Source: CAD feature listing. Evaluate the final solid. Frame: model axes, mm. A direction names the side the tool comes from. Coordinates: 2 decimals unless noted, no trailing zeros. Order: outer loops, then holes, each group sorted by start corner. A loop starts at its lowest first (then second) coordinate and runs counter-clockwise, first axis right, second up.
```python
from build123d import *

# Parameters (mm, degrees)
SALIENTE_EXTRUIR1_DEPTH = 3


with BuildPart() as part:
    # Croquis1 → Saliente-Extruir1 (new body)
    with BuildSketch(Plane.XY):
        with BuildLine():
            ThreePointArc((-9.805994702, 4.781775998), (-9.445994702, 4.421775998), (-9.445994702, 3.912659116))
            ThreePointArc((-9.445994702, 3.912659116), (-9.805994702, 3.552659116), (-10.315111585, 3.552659116))
            Line((-10.315111585, 3.552659116), (-14.665897198, 5.354813524))
            Line((-14.665897198, 5.354813524), (-14.942220541, 4.584446936))
            ThreePointArc((-14.942220541, 4.584446936), (-13.141116636, 2.599696402), (-12.489358574, 0))
            ThreePointArc((-12.489358574, 0), (-13.40224475, -3.037731981), (-15.838448045, -5.06900997))
            ThreePointArc((-15.838448045, -5.06900997), (-15.725960944, -5.407906335), (-15.606223383, -5.744309383))
            Line((-15.606223383, -5.744309383), (-10.315111585, -3.552659116))
            ThreePointArc((-10.315111585, -3.552659116), (-9.445994702, -3.912659116), (-9.805994702, -4.781775998))
            Line((-9.805994702, -4.781775998), (-15.0971065, -6.973426265))
            ThreePointArc((-15.0971065, -6.973426265), (-14.943900866, -7.295966383), (-14.78380534, -7.615142693))
            ThreePointArc((-14.78380534, -7.615142693), (-9.642639792, -8.161938898), (-7.217280635, -12.727922061))
            ThreePointArc((-7.217280635, -12.727922061), (-7.317660389, -13.774935704), (-7.615142693, -14.78380534))
            ThreePointArc((-7.615142693, -14.78380534), (-7.295966383, -14.943900866), (-6.973426265, -15.0971065))
            Line((-6.973426265, -15.0971065), (-4.781775998, -9.805994702))
            ThreePointArc((-4.781775998, -9.805994702), (-3.912659116, -9.445994702), (-3.552659116, -10.315111585))
            Line((-3.552659116, -10.315111585), (-5.744309383, -15.606223383))
            ThreePointArc((-5.744309383, -15.606223383), (-5.407906335, -15.725960944), (-5.06900997, -15.838448045))
            ThreePointArc((-5.06900997, -15.838448045), (0, -12.489358574), (5.06900997, -15.838448045))
            ThreePointArc((5.06900997, -15.838448045), (5.407906335, -15.725960944), (5.744309383, -15.606223383))
            Line((5.744309383, -15.606223383), (3.552659116, -10.315111585))
            ThreePointArc((3.552659116, -10.315111585), (3.912659116, -9.445994702), (4.781775998, -9.805994702))
            Line((4.781775998, -9.805994702), (6.973426265, -15.0971065))
            ThreePointArc((6.973426265, -15.0971065), (7.295966383, -14.943900866), (7.615142693, -14.78380534))
            ThreePointArc((7.615142693, -14.78380534), (8.83131014, -8.83131014), (14.78380534, -7.615142693))
            ThreePointArc((14.78380534, -7.615142693), (14.943900866, -7.295966383), (15.0971065, -6.973426265))
            Line((15.0971065, -6.973426265), (9.805994702, -4.781775998))
            ThreePointArc((9.805994702, -4.781775998), (9.445994702, -3.912659116), (10.315111585, -3.552659116))
            Line((10.315111585, -3.552659116), (15.606223383, -5.744309383))
            ThreePointArc((15.606223383, -5.744309383), (15.725960944, -5.407906335), (15.838448045, -5.06900997))
            ThreePointArc((15.838448045, -5.06900997), (12.489358574, 0), (15.838448045, 5.06900997))
            ThreePointArc((15.838448045, 5.06900997), (15.725960944, 5.407906335), (15.606223383, 5.744309383))
            Line((15.606223383, 5.744309383), (10.315111585, 3.552659116))
            ThreePointArc((10.315111585, 3.552659116), (9.445994702, 3.912659116), (9.805994702, 4.781775998))
            Line((9.805994702, 4.781775998), (15.0971065, 6.973426265))
            ThreePointArc((15.0971065, 6.973426265), (14.943900866, 7.295966383), (14.78380534, 7.615142693))
            ThreePointArc((14.78380534, 7.615142693), (8.83131014, 8.83131014), (7.615142693, 14.78380534))
            ThreePointArc((7.615142693, 14.78380534), (7.295966383, 14.943900866), (6.973426265, 15.0971065))
            Line((6.973426265, 15.0971065), (4.781775998, 9.805994702))
            ThreePointArc((4.781775998, 9.805994702), (3.912659116, 9.445994702), (3.552659116, 10.315111585))
            Line((3.552659116, 10.315111585), (5.744309383, 15.606223383))
            ThreePointArc((5.744309383, 15.606223383), (5.407906335, 15.725960944), (5.06900997, 15.838448045))
            ThreePointArc((5.06900997, 15.838448045), (0, 12.489358574), (-5.06900997, 15.838448045))
            ThreePointArc((-5.06900997, 15.838448045), (-5.407906335, 15.725960944), (-5.744309383, 15.606223383))
            Line((-5.744309383, 15.606223383), (-3.552659116, 10.315111585))
            ThreePointArc((-3.552659116, 10.315111585), (-3.912659116, 9.445994702), (-4.781775998, 9.805994702))
            Line((-4.781775998, 9.805994702), (-6.973426265, 15.0971065))
            ThreePointArc((-6.973426265, 15.0971065), (-7.295966383, 14.943900866), (-7.615142693, 14.78380534))
            ThreePointArc((-7.615142693, 14.78380534), (-7.317660389, 13.774935704), (-7.217280635, 12.727922061))
            ThreePointArc((-7.217280635, 12.727922061), (-9.642639792, 8.161938898), (-14.78380534, 7.615142693))
            ThreePointArc((-14.78380534, 7.615142693), (-14.870201448, 7.445025684), (-14.954640105, 7.273928642))
            ThreePointArc((-14.954640105, 7.273928642), (-14.628849784, 7.038643274), (-14.422305364, 6.693914482))
            Line((-14.422305364, 6.693914482), (-9.805994702, 4.781775998))
        make_face()
        with BuildLine():
            ThreePointArc((0.665193263, 0), (-0.129772768, -0.652411761), (-0.614558441, 0.254558441))
            ThreePointArc((-0.614558441, 0.254558441), (0.129772768, 0.652411761), (0.665193263, 0))
        make_face(mode=Mode.SUBTRACT)
    extrude(amount=-SALIENTE_EXTRUIR1_DEPTH)


solid = part.part
```
Q1. Material intervals for line 1 along X through (y, z) = (-10.5, -1.95); line 2 along Y through (x, z) = (-5, -2.55); line 3 along Y through (x, z) = (-0.5, -2.05), sorted ascending.
Solutions:
line 1: x = -7.69 to -5.07, -3.63 to 3.63, 5.07 to 7.69
line 2: y = -15.68 to -13.81, -10.33 to 10.33, 13.81 to 15.68
line 3: y = -12.51 to -0.44, 0.44 to 12.51
Q2. Section query B-B on y = -13.5. Output: boundary loops of the cut face in (x, z), plus the area to 3 significant figures.
Solutions:
outline: (-7.27, -3) - (-6.31, -3) - (-6.31, 0) - (-7.27, 0) - close; (-4.87, -3) - (-3.18, -3) - (-3.18, 0) - (-4.87, 0) - close; (3.18, -3) - (4.87, -3) - (4.87, 0) - (3.18, 0) - close; (6.31, -3) - (7.27, -3) - (7.27, 0) - (6.31, 0) - close
area: 15.9 mm2
Q3. Pin query (flat end, axial travel): P1, Ø1.5, axis at x = 3, z = -2, coming from the +Y side; P2, Ø0.8, axis at x = 0, y = 0, coming from the -Z side; P3, Ø1.5, axis at y = -10.5, z = -2.5, coming from the +X side; P4, Ø1, axis at x = -2.5, z = -1.5, coming from the +Y side. Return the tip coordinate at first contact, or that it passes through.
Solutions:
P1: stops at y = 13.96
P2: passes through
P3: stops at x = 8.09
P4: stops at y = 13.38
Q4. Section query A-A on x = 0. Output: boundary loops of the cut face in (y, z).
Solutions:
outline: (-12.49, -3) - (-0.67, -3) - (-0.67, 0) - (-12.49, 0) - close; (0.67, -3) - (12.49, -3) - (12.49, 0) - (0.67, 0) - close
Q5. Set-up query: faces 1 (the flat face through (4.63, 12.92, -1.48)), 2 (the cylindrical face through (-0.09, -12.49, -1.48)). Return all of +Z, -Z, +X, -X, +Y, -Y with unobstructed straight access to the full face (end or side cutting, diameter ignored); none if empty.
Solutions:
face 1: +Z, -Z
face 2: +Z, -Z, -Y
Q6. Pull-direction query (X, two-part tool) for faces 3 (the cylindrical face through (12.49, -0.09, -1.48)), 4 (the flat face through (5.86, -12.41, -1.48)); classes: pulls with the +X half, pulls with the -X half, needs draft (parallel to the pull), parting line crosses it, or undercut.
Solutions:
face 3: pulls with the +X half
face 4: undercut
Q7. Section query C-C on y = 11. Output: boundary loops of the cut face in (x, z).
Solutions:
outline: (-7.5, -3) - (-5.28, -3) - (-5.28, 0) - (-7.5, 0) - close; (-3.84, -3) - (3.84, -3) - (3.84, 0) - (-3.84, 0) - close; (5.28, -3) - (7.5, -3) - (7.5, 0) - (5.28, 0) - close
